CAD build for the part. Positions are in the model's coordinates, mm. A direction names the side the tool comes from. Give positions to 0.01 mm unless a question says otherwise; leave off trailing zeros. Loops run counter-clockwise (first coordinate to the right, second up) from the corner with the lowest first, then second, coordinate; pieces in that order, holes last. Notation, with made-up numbers: M -35.5,62 L -30.5,62 A30 ccw -30.5,96 Z; hole C 49,-30 d2. An arc over 180 degrees is marked long. One line per question, with ' | ' between items.
```python
from build123d import *

# Parameters (mm, degrees)
SKETCH1_R           = 50
BOSS_EXTRUDE1_DEPTH = 30
FILLET1_R           = 10
SKETCH2_R           = 40
CUT_EXTRUDE1_DEPTH  = 10
CUT_EXTRUDE2_START  = -10
SKETCH3_R           = 40
CUT_EXTRUDE2_DEPTH  = 10
SCALE1_SCALE        = 2


with BuildPart() as part:
    # Sketch1 → Boss-Extrude1 (new body)
    with BuildSketch(Plane.XY):
        Circle(SKETCH1_R)
    extrude(amount=BOSS_EXTRUDE1_DEPTH)

    # Fillet1
    fillet1_edges = [part.edges().sort_by_distance(p)[0] for p in [
        (-50, 0, 0),
        (-50, 0, 30),
    ]]
    fillet(fillet1_edges, radius=FILLET1_R)

    # Sketch2 → Cut-Extrude1 (cut)
    with BuildSketch(Plane.XY.offset(30)):
        Circle(SKETCH2_R)
    extrude(amount=-CUT_EXTRUDE1_DEPTH, mode=Mode.SUBTRACT)

    # Sketch3 → Cut-Extrude2 (cut)
    with BuildSketch(Plane(origin=(0, 0, 0), x_dir=(-1, 0, 0), z_dir=(0, 0, -1)).offset(CUT_EXTRUDE2_START)):
        with Locations(Location((0, 0, 0), (0, 0, 180))):
            Circle(SKETCH3_R)
    extrude(amount=CUT_EXTRUDE2_DEPTH, mode=Mode.SUBTRACT)


with BuildPart() as part_1:
    # Scale1: scaled about (0, 0, 15)
    add(part.part.scale(SCALE1_SCALE).moved(Location((0, 0, -15))))


solid = part_1.part
```
Item 1: Saw through at D-D on z = 28.5. Give the cut face in (x, y), and give its area (3 significant figures).
Conclusion:
outline: C 0,0 d199.38; hole C 0,0 d160 | area: 11,100 mm²
Item 2: Saw through at C-C on z = 16. Give the cut face in (x, y).
Conclusion:
outline: C 0,0 d200
Item 3: Drill centre lines: line 1 along Z through (x, y) = (61.5, -6); line 2 along Y through (x, z) = (56.5, -3); line 3 along Y through (x, z) = (0, 32) (3 decimals). Where is each one in solid material? Low to high. Write a range as [from, to].
Conclusion:
line 1: [5, 25] | line 2: [-80.48, -56.64], [56.64, 80.48] | line 3: [-98.735, -80], [80, 98.735]
Item 4: 3-axis set-ups, long thin cutter, end or side, ignore diameter. For faces 3 (the cylindrical face through (-17.34, -78.1, 35.14)), 4 (the flat face through (-1, -1, 5)): which of +Z, -Z, +X, -X, +Y, -Y reach the whole face in a straight line?
Conclusion:
face 3: +Z | face 4: -Z
Item 5: Mould opens along Y. For faces 1 (the cylindrical face through (95.38, 30.04, 14.86)), 2 (the flat face through (-1, 1, 25)) say: pulls with the +Y half, pulls with the -Y half, needs draft (parallel to the pull), parting line crosses it, or undercut.
Conclusion:
face 1: parting line crosses it | face 2: undercut
Item 6: Drop flat-ended pins along their axis: P1, Ø12, axis at y = 56, z = 28, coming from the -X side; P2, Ø3, axis at x = -8.5, y = 3, coming from the +Z side; P3, Ø3, axis at x = 28, z = 5.5, coming from the -Y side. Give the stop position or say it passes through.
Conclusion:
P1: x = -86.44 | P2: z = 25 | P3: y = -96.42
Item 7: Saw through at A-A on x = 0. Give the cut face in (y, z).
Conclusion:
outline: M -100,5 A20 ccw -80,-15 L -80,5 L 80,5 L 80,-15 A20 ccw 100,5 L 100,25 A20 ccw 80,45 L 80,25 L -80,25 L -80,45 A20 ccw -100,25 Z
